Could you check a few things on this model? Use its own coordinates, in mm. Face numbers are marked on the shaded views. A direction names the side the tool comes from. Coordinates: 2 decimals unless noted, no trailing zeros. Loops run counter-clockwise (first coordinate to the right, second up) from the corner with the lowest first, then second, coordinate; pieces in that order, holes last.
1) Imagine slicing it at B-B on z = -55.5. Please give me the cut outline in (x, y), plus the area to 3 significant figures.
2) Imagine slicing it at D-D on y = -18. Please give me the cut outline in (x, z), plus the area to 3 significant figures.
3) For the marked faces 4, 5 and 6, which set-ups out of +Z, -Z, +X, -X, +Y, -Y let a thin tool reach every point of the face, with its end or its side?
4) Will these pins go through, and if not, where does the flat tip stop? P1, Ø10, axis at x = -87.5, y = -1.5, coming from the +Z side; P2, Ø1.5, axis at y = -1, z = -59.5, coming from the -X side; P3, Ø1, axis at x = -73.5, y = -6.5, coming from the +Z side.
5) Imagine slicing it at A-A on y = 12. Please give me the cut outline in (x, z).
6) If I drill on line 1 along Y through (x, z) = (-77, -46.5); line 2 along Y through (x, z) = (-78.5, -113.5); line 3 along X through (y, z) = (-1.5, -105), over which ranges is the centre line in solid material (lowest first)?
7) Imagine slicing it at C-C on x = -71.5. Please give me the cut outline in (y, z).
8) Thinking about a two-plate mould opening in X: for the marked faces 1, 2 and 3, which applies, released by +X, released by -X, zero draft, split by the parting line, or undercut?
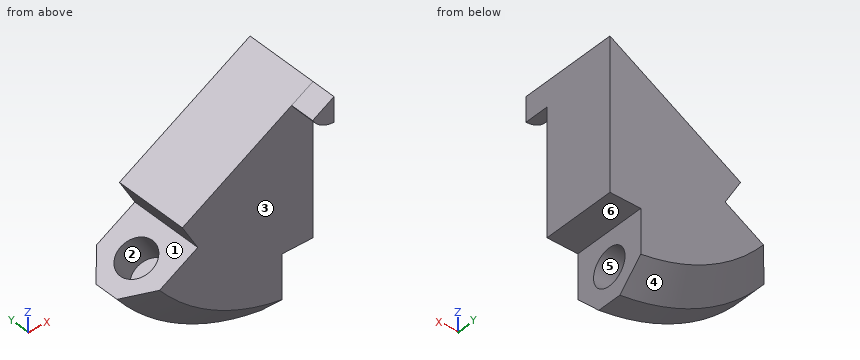
```python
from build123d import *

# Parameters (mm, degrees)
SALIENTE_EXTRUIR1_DEPTH = 15
CORTAR_EXTRUIR2_DEPTH   = 30
CROQUIS4_R              = 7.5
CORTAR_EXTRUIR3_DEPTH   = 13
CROQUIS5_R              = 7.5
CORTAR_EXTRUIR4_DEPTH   = 13
SALIENTE_EXTRUIR2_DEPTH = 10
CHAFL_N1_SIZE           = 10
CHAFL_N2_SIZE           = 10


with BuildPart() as part:
    # Croquis1 → Saliente-Extruir1 (new, symmetric)
    with BuildSketch(Plane(origin=(0, 0, 0), x_dir=(1, 0, 0), z_dir=(0, 1, 0))):
        with BuildLine():
            Line((-136.742226614, -20.094724465), (-112.493515308, -6.094724465))
            Line((-112.493515308, -6.094724465), (-118.743515308, 4.730593082))
            Line((-118.743515308, 4.730593082), (-124.993515308, 15.55591063))
            Line((-124.993515308, 15.55591063), (-149.242226614, 1.55591063))
            ThreePointArc((-149.242226614, 1.55591063), (-155.805359207, 35.294451757), (-149.242226614, 69.032992885))
            Line((-149.242226614, 69.032992885), (-124.993515308, 55.032992885))
            Line((-124.993515308, 55.032992885), (-118.743515308, 65.858310432))
            Line((-118.743515308, 65.858310432), (-112.493515308, 76.68362798))
            Line((-112.493515308, 76.68362798), (-136.742226614, 90.68362798))
            ThreePointArc((-136.742226614, 90.68362798), (-110.805359207, 113.236738098), (-78.305359207, 124.422169107))
            Line((-78.305359207, 124.422169107), (-78.305359207, 96.422169107))
            Line((-78.305359207, 96.422169107), (-65.805359207, 96.422169107))
            Line((-65.805359207, 96.422169107), (-53.305359207, 96.422169107))
            Line((-53.305359207, 96.422169107), (-53.305359207, 124.422169107))
            ThreePointArc((-53.305359207, 124.422169107), (-20.805359207, 113.236738098), (5.131508199, 90.68362798))
            Line((5.131508199, 90.68362798), (-19.117203107, 76.68362798))
            Line((-19.117203107, 76.68362798), (-6.617203107, 55.032992885))
            Line((-6.617203107, 55.032992885), (17.631508199, 69.032992885))
            ThreePointArc((17.631508199, 69.032992885), (24.194640793, 35.294451757), (17.631508199, 1.55591063))
            Line((17.631508199, 1.55591063), (-6.617203107, 15.55591063))
            Line((-6.617203107, 15.55591063), (-12.867203107, 4.730593082))
            Line((-12.867203107, 4.730593082), (-19.117203107, -6.094724465))
            Line((-19.117203107, -6.094724465), (5.131508199, -20.094724465))
            ThreePointArc((5.131508199, -20.094724465), (-20.805359207, -42.647834583), (-53.305359207, -53.833265593))
            Line((-53.305359207, -53.833265593), (-53.305359207, -25.833265593))
            Line((-53.305359207, -25.833265593), (-65.805359207, -25.833265593))
            Line((-65.805359207, -25.833265593), (-78.305359207, -25.833265593))
            Line((-78.305359207, -25.833265593), (-78.305359207, -53.833265593))
            ThreePointArc((-78.305359207, -53.833265593), (-110.805359207, -42.647834583), (-136.742226614, -20.094724465))
        make_face()
    extrude(amount=SALIENTE_EXTRUIR1_DEPTH, both=True)

    # Croquis3 → Cortar-Extruir2 (cut)
    with BuildSketch(Plane(origin=(0, 15, 0), x_dir=(1, 0, 0), z_dir=(0, 1, 0))):
        with BuildLine():
            Line((-65.805359207, 96.422169107), (-65.805359207, 35.294451757))
            Line((-65.805359207, 35.294451757), (-118.743515308, 65.858310432))
            Line((-118.743515308, 65.858310432), (-112.493515308, 76.68362798))
            Line((-112.493515308, 76.68362798), (-136.742226614, 90.68362798))
            ThreePointArc((-136.742226614, 90.68362798), (-20.805359207, -42.647834583), (-78.305359207, 124.422169107))
            Line((-78.305359207, 124.422169107), (-78.305359207, 96.422169107))
            Line((-78.305359207, 96.422169107), (-65.805359207, 96.422169107))
        make_face()
    extrude(amount=-CORTAR_EXTRUIR2_DEPTH, mode=Mode.SUBTRACT)

    # Croquis4 → Cortar-Extruir3 (cut)
    with BuildSketch(Plane(origin=(-78.305359207, 0, 0), x_dir=(0, 0, -1), z_dir=(1, 0, 0))):
        with Locations((110.422169107, 0)):
            Circle(CROQUIS4_R)
    extrude(amount=-CORTAR_EXTRUIR3_DEPTH, mode=Mode.SUBTRACT)

    # Croquis5 → Cortar-Extruir4 (cut)
    with BuildSketch(Plane(origin=(5.081606115, 0, -8.801599976), x_dir=(0.8660254037844403, 0, 0.4999999999999971), z_dir=(-0.49999999999999717, 0, 0.8660254037844404))):
        with Locations((-149.764056007, 0)):
            Circle(CROQUIS5_R)
    extrude(amount=-CORTAR_EXTRUIR4_DEPTH, mode=Mode.SUBTRACT)

    # Croquis6 → Saliente-Extruir2 (add)
    with BuildSketch(Plane.XZ.offset(15)):
        with BuildLine():
            Line((-65.805359207, -35.294451757), (-74.465613245, -40.294451757))
            ThreePointArc((-74.465613245, -40.294451757), (-70.805359207, -43.954705795), (-65.805359207, -45.294451757))
            Line((-65.805359207, -45.294451757), (-65.805359207, -35.294451757))
        make_face()
    extrude(amount=SALIENTE_EXTRUIR2_DEPTH)

    # Chaflán1
    chafl_n1_edges = [part.edges().sort_by_distance(p)[0] for p in [
        (-110.805359207, -15, -113.236738098),
    ]]
    chamfer(chafl_n1_edges, length=CHAFL_N1_SIZE)

    # Chaflán2
    chafl_n2_edges = [part.edges().sort_by_distance(p)[0] for p in [
        (-110.805359207, 15, -113.236738098),
    ]]
    chamfer(chafl_n2_edges, length=CHAFL_N2_SIZE)


solid = part.part
```
Filled in:
1. outline: (-100.8, -15) - (-65.81, -15) - (-65.81, 15) - (-100.8, 15) - close
1. area: 1,050 mm2
2. outline: (-74.47, -40.29) arc R10 ccw to (-65.81, -45.29) - (-65.81, -35.29) - close
2. area: 52.4 mm2
3. face 4: -Z, -X, +Y
3. face 5: +X
3. face 6: -Z, +X, +Y, -Y
4. P1: stops at z = -44.93
4. P2: stops at x = -109.03
4. P3: stops at z = -39.45
5. outline: (-130.62, -87.15) arc R83 ccw to (-78.31, -117.35) - (-78.31, -96.42) - (-65.81, -96.42) - (-65.81, -35.29) - (-118.74, -65.86) - (-112.49, -76.68) - close
6. line 1: y = -15 to 15
6. line 2: y = -15 to -6.84, 6.84 to 15
6. line 3: x = -122.74 to -91.31
7. outline: (-25, -43.51) - (-15, -43.51) - (-15, -96.42) - (15, -96.42) - (15, -38.58) - (-25, -38.58) - close
8. face 1: released by -X
8. face 2: undercut
8. face 3: zero draft
